The listing builds one solid part. Answer for the finished solid, in the listing's coordinates (mm). Coordinates: 2 decimals unless noted, no trailing zeros. Order: outer loops, then holes, each group sorted by start corner. A loop starts at its lowest first (then second) coordinate and runs counter-clockwise, first axis right, second up.
```python
from build123d import *

# Parameters (mm, degrees)
ESQUISSE1_W             = 295
ESQUISSE1_H             = 260
BOSS_EXTRU_1_DEPTH      = 5
ESQUISSE3_OUTSIDE_W     = 375.652
ESQUISSE3_OUTSIDE_H     = 340.652
ESQUISSE3_OUTSIDE_W_2   = 264.6
ESQUISSE3_OUTSIDE_H_2   = 200
ENL_V_MAT_EXTRU_2_DEPTH = 394.255642045
CONG_1_R                = 100
ENL_V_MAT_EXTRU_4_DEPTH = 363.233405417
ESQUISSE7_W             = 123.401082374
ESQUISSE7_H             = 15
ENL_V_MAT_EXTRU_6_DEPTH = 363.233405417


with BuildPart() as part:
    # Esquisse1 → Boss.-Extru.1 (new body)
    with BuildSketch(Plane.XY):
        with Locations((-147.5, -130)):
            Rectangle(ESQUISSE1_W, ESQUISSE1_H)
    extrude(amount=BOSS_EXTRU_1_DEPTH)

    # Esquisse3 outside → Enlèv. mat.-Extru.2 (cut, through all)
    with BuildSketch(Plane(origin=(0, 0, 0), x_dir=(-1, 0, 0), z_dir=(0, 0, -1))):
        with Locations((147.5, -130)):
            Rectangle(ESQUISSE3_OUTSIDE_W, ESQUISSE3_OUTSIDE_H)
        with Locations((147.5, -130)):
            Rectangle(ESQUISSE3_OUTSIDE_W_2, ESQUISSE3_OUTSIDE_H_2, mode=Mode.SUBTRACT)
    extrude(amount=-ENL_V_MAT_EXTRU_2_DEPTH, mode=Mode.SUBTRACT)

    # Congé1
    cong_1_edges = [part.edges().sort_by_distance(p)[0] for p in [
        (-279.8, -30, 2.5),
        (-15.2, -30, 2.5),
        (-279.8, -230, 2.5),
        (-15.2, -230, 2.5),
    ]]
    fillet(cong_1_edges, radius=CONG_1_R - 0.0001)  # a hair under: the kernel refuses the full size

    # Esquisse5 → Enlèv. mat.-Extru.4 (cut, through all)
    with BuildSketch(Plane.XY.offset(5)):
        with BuildLine():
            ThreePointArc((-70.799458813, -198.530608435), (-73.627885938, -199.70218131), (-74.799458813, -202.530608435))
            Line((-74.799458813, -202.530608435), (-70.799458813, -202.530608435))
            Line((-70.799458813, -202.530608435), (-70.799458813, -198.530608435))
        make_face()
        with BuildLine():
            Line((-70.799458813, -202.530608435), (-74.799458813, -202.530608435))
            ThreePointArc((-74.799458813, -202.530608435), (-70.799458813, -206.530608435), (-66.799458813, -202.530608435))
            ThreePointArc((-66.799458813, -202.530608435), (-67.971031689, -199.70218131), (-70.799458813, -198.530608435))
            Line((-70.799458813, -198.530608435), (-70.799458813, -202.530608435))
        make_face()
        with BuildLine():
            ThreePointArc((-224.200541187, -198.530608435), (-227.028968311, -205.35903556), (-220.200541187, -202.530608435))
            Line((-220.200541187, -202.530608435), (-224.200541187, -202.530608435))
            Line((-224.200541187, -202.530608435), (-224.200541187, -198.530608435))
        make_face()
        with BuildLine():
            Line((-224.200541187, -202.530608435), (-220.200541187, -202.530608435))
            ThreePointArc((-220.200541187, -202.530608435), (-221.372114062, -199.70218131), (-224.200541187, -198.530608435))
            Line((-224.200541187, -198.530608435), (-224.200541187, -202.530608435))
        make_face()
        with BuildLine():
            ThreePointArc((-220.200541187, -72.530608435), (-227.028968311, -69.70218131), (-224.200541187, -76.530608435))
            Line((-224.200541187, -76.530608435), (-224.200541187, -72.530608435))
            Line((-224.200541187, -72.530608435), (-220.200541187, -72.530608435))
        make_face()
        with BuildLine():
            Line((-224.200541187, -72.530608435), (-224.200541187, -76.530608435))
            ThreePointArc((-224.200541187, -76.530608435), (-221.372114062, -75.35903556), (-220.200541187, -72.530608435))
            Line((-220.200541187, -72.530608435), (-224.200541187, -72.530608435))
        make_face()
        with BuildLine():
            ThreePointArc((-74.799458813, -72.530608435), (-73.627885938, -75.35903556), (-70.799458813, -76.530608435))
            Line((-70.799458813, -76.530608435), (-70.799458813, -72.530608435))
            Line((-70.799458813, -72.530608435), (-74.799458813, -72.530608435))
        make_face()
        with BuildLine():
            Line((-70.799458813, -72.530608435), (-70.799458813, -76.530608435))
            ThreePointArc((-70.799458813, -76.530608435), (-67.971031689, -75.35903556), (-66.799458813, -72.530608435))
            ThreePointArc((-66.799458813, -72.530608435), (-70.799458813, -68.530608435), (-74.799458813, -72.530608435))
            Line((-74.799458813, -72.530608435), (-70.799458813, -72.530608435))
        make_face()
    extrude(amount=-ENL_V_MAT_EXTRU_4_DEPTH, mode=Mode.SUBTRACT)

    # Esquisse7 → Enlèv. mat.-Extru.6 (cut, through all)
    with BuildSketch(Plane(origin=(0, 0, 0), x_dir=(-1, 0, 0), z_dir=(0, 0, -1))):
        with Locations((147.5, -67.5)):
            Rectangle(ESQUISSE7_W, ESQUISSE7_H)
        with Locations((147.5, -192.5)):
            Rectangle(ESQUISSE7_W, ESQUISSE7_H)
    extrude(amount=-ENL_V_MAT_EXTRU_6_DEPTH, mode=Mode.SUBTRACT)


solid = part.part
```
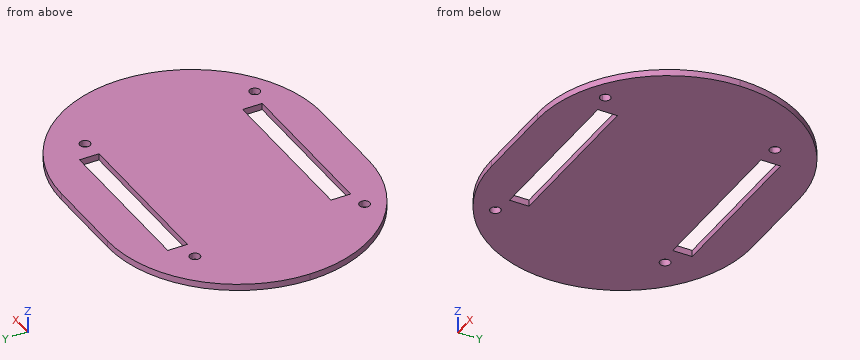
1) A cutting plane is placed at A-A, the plane x = -151. Write down the section's boundary in (y, z), plus the area to 3 significant figures.
2) Straight lines are drawn through the part: probe 1 along Y at (x, z) = (-122, 2.05); probe 2 along Y at (x, z) = (-110, 4.5); probe 3 along X at (y, z) = (-72, 2.1). For each, find the intervals that lie inside material, in ascending order.
3) A cutting plane is placed at C-C, the plane x = -107.5. Write down the section's boundary in (y, z), plus the area to 3 significant figures.
4) A cutting plane is placed at B-B, the plane z = 4.05. Count the separate pieces of the cut face and the enclosed holes in it, plus the area to 3 significant figures.
5) A cutting plane is placed at D-D, the plane y = -170.5. Write down the section's boundary in (x, z), plus the area to 3 significant figures.
6) Each of these flat-tipped pins is pushed along its axis until it touches: P1, Ø3, axis at y = -146, z = 2.5, coming from the +X side; P2, Ø1.5, axis at x = -148, y = -182.5, coming from the -Z side; P3, Ø2.5, axis at y = -71, z = 3, coming from the +X side; P4, Ø2, axis at x = -240.5, z = 1.5, coming from the -Y side. Where does it stop, or does it pass through?
Working result:
1. outline: (-230, 0) - (-200, 0) - (-200, 5) - (-230, 5) - close; (-185, 0) - (-75, 0) - (-75, 5) - (-185, 5) - close; (-60, 0) - (-30, 0) - (-30, 5) - (-60, 5) - close
1. area: 850 mm2
2. probe 1: y = -230 to -200, -185 to -75, -60 to -30
2. probe 2: y = -229.86 to -200, -185 to -75, -60 to -30.14
2. probe 3: x = -261.26 to -228.17, -220.24 to -209.2, -85.8 to -74.76, -66.83 to -33.74
3. outline: (-229.7, 0) - (-200, 0) - (-200, 5) - (-229.7, 5) - close; (-185, 0) - (-75, 0) - (-75, 5) - (-185, 5) - close; (-60, 0) - (-30.3, 0) - (-30.3, 5) - (-60, 5) - close
3. area: 847 mm2
4. separate pieces: 1
4. enclosed holes: 6
4. area: 40,400 mm2
5. outline: (-271.23, 0) - (-23.77, 0) - (-23.77, 5) - (-271.23, 5) - close
5. area: 1,240 mm2
6. P1: stops at x = -16.26
6. P2: stops at z = 0
6. P3: stops at x = -33.56
6. P4: stops at y = -210.22
